CAD build for the part. Positions are in the model's coordinates, mm. Face numbers are marked on the shaded views. A direction names the side the tool comes from. Round coordinates to 2 decimals unless told otherwise and drop trailing zeros. Loops run counter-clockwise (first coordinate to the right, second up) from the corner with the lowest first, then second, coordinate; pieces in that order, holes last. Notation, with made-up numbers: (-21, -26.75) -> (11, -26.75) arc R27 ccw to (11, -9.75) -> close; hole circle Ø3 at (67.5, -8). An arc over 180 degrees is marked (long way). Answer as CSV lines item,"result".
```python
from build123d import *

# Parameters (mm, degrees)
SKETCH1_W                = 42.418
SKETCH1_H                = 0.006053875
SKETCH1_H_2              = 42.424053875
BOSS_EXTRUDE1_DEPTH      = 58.42
CUT_EXTRUDE3_DEPTH       = 68.58
SKETCH3_W                = 38.1
SKETCH3_H                = 15.367
SKETCH3_W_2              = 76.2
CUT_EXTRUDE4_DEPTH       = 77.078788463
BOSS_EXTRUDE6_DEPTH      = 3.302
BOSS_EXTRUDE6_DEPTH_BACK = 60
CUT_EXTRUDE9_DEPTH       = 106
SKETCH4_R                = 2.667
CUT_EXTRUDE6_DEPTH       = 106
CUT_EXTRUDE6_DEPTH_BACK  = 20
CUT_EXTRUDE13_DEPTH      = 106
SKETCH11_R               = 35
CUT_EXTRUDE15_DEPTH      = 106


with BuildPart() as part:
    # Sketch1 → Boss-Extrude1 (new body)
    with BuildSketch(Plane(origin=(0, 0, 0), x_dir=(1, 0, 0), z_dir=(0, 1, 0))):
        with BuildLine():
            ThreePointArc((36.658549334, 5.015053409), (0, 37), (-36.658549334, 5.015053409))
            Line((-36.658549334, 5.015053409), (-25.85615018, -105.598244919))
            ThreePointArc((-25.85615018, -105.598244919), (0, -129.052312238), (25.85615018, -105.598244919))
            Line((25.85615018, -105.598244919), (36.658549334, 5.015053409))
        make_face()
        with Locations((0, 21.205973063)):
            Rectangle(SKETCH1_W, SKETCH1_H, mode=Mode.SUBTRACT)
        with Locations((0, -21.212026937)):
            Rectangle(SKETCH1_W, SKETCH1_H, mode=Mode.SUBTRACT)
        with Locations((0, -45.723026938)):
            Rectangle(SKETCH1_W, SKETCH1_H_2, mode=Mode.SUBTRACT)
    extrude(amount=BOSS_EXTRUDE1_DEPTH)

    # Sketch2 → Cut-Extrude3 (cut)
    with BuildSketch(Plane(origin=(0, 58.42, 0), x_dir=(1, 0, 0), z_dir=(0, 1, 0))):
        with BuildLine():
            Line((-21.209, -66.935053875), (-17.681227978, -103.058371806))
            ThreePointArc((-17.681227978, -103.058371806), (0, -119.096981901), (17.681227978, -103.058371806))
            Line((17.681227978, -103.058371806), (21.209, -66.935053875))
            Line((21.209, -66.935053875), (-21.209, -66.935053875))
        make_face()
    extrude(amount=-CUT_EXTRUDE3_DEPTH, mode=Mode.SUBTRACT)

    # Sketch3 → Cut-Extrude4 (cut, through all)
    with BuildSketch(Plane(origin=(35.827089604, 0, 3.498842619), x_dir=(0.097196738, 0, -0.995265188), z_dir=(0.995265188, 0, 0.097196738))):
        with Locations((-121.635123595, 7.6835)):
            Rectangle(SKETCH3_W, SKETCH3_H)
        with Locations((-83.535123595, 7.6835)):
            Rectangle(SKETCH3_W, SKETCH3_H)
        with Locations((-102.585123595, 50.7365)):
            Rectangle(SKETCH3_W_2, SKETCH3_H)
    extrude(amount=-CUT_EXTRUDE4_DEPTH, mode=Mode.SUBTRACT)

    # Sketch7 → Boss-Extrude6 (add, two sides)
    with BuildSketch(Plane.XY.offset(21.209)) as boss_extrude6_sk:
        with BuildLine():
            Line((-34.93, 93.35), (-40.014696591, 94.207479888))
            Line((-40.014696591, 94.207479888), (-40.014696591, 55.40139672))
            Line((-40.014696591, 55.40139672), (41.480417685, 55.40139672))
            Line((41.480417685, 55.40139672), (41.480417685, 93.35))
            Line((41.480417685, 93.35), (34.93, 93.35))
            ThreePointArc((34.93, 93.35), (0, 58.42), (-34.93, 93.35))
        make_face()
    extrude(amount=BOSS_EXTRUDE6_DEPTH)
    extrude(boss_extrude6_sk.sketch, amount=-BOSS_EXTRUDE6_DEPTH_BACK)

    # Sketch9 → Cut-Extrude9 (cut)
    with BuildSketch(Plane.XZ):
        with BuildLine():
            Line((36.658549334, -5.015053409), (29.559345914, 67.678641264))
            Line((29.559345914, 67.678641264), (73.660631966, -15.324129582))
            Line((73.660631966, -15.324129582), (14.272065625, -84.211573711))
            Line((14.272065625, -84.211573711), (-60.028569558, -39.869360469))
            Line((-60.028569558, -39.869360469), (-30.128608249, 61.849567226))
            Line((-30.128608249, 61.849567226), (-36.658549334, -5.015053409))
            ThreePointArc((-36.658549334, -5.015053409), (0, -37), (36.658549334, -5.015053409))
        make_face()
    extrude(amount=-CUT_EXTRUDE9_DEPTH, mode=Mode.SUBTRACT)

    # Sketch4 → Cut-Extrude6 (cut, two sides)
    with BuildSketch(Plane(origin=(0, 58.42, 0), x_dir=(1, 0, 0), z_dir=(0, 1, 0))) as cut_extrude6_sk:
        with Locations((9.8, 0.389)):
            Circle(SKETCH4_R)
    extrude(amount=CUT_EXTRUDE6_DEPTH, mode=Mode.SUBTRACT)
    extrude(cut_extrude6_sk.sketch, amount=-CUT_EXTRUDE6_DEPTH_BACK, mode=Mode.SUBTRACT)

    # Sketch10 → Cut-Extrude13 (cut)
    with BuildSketch(Plane(origin=(35.827089604, 0, 3.498842619), x_dir=(0.097196738, 0, -0.995265188), z_dir=(0.995265188, 0, 0.097196738))):
        Polygon((-21.112119301, 84.442127612), (-21.112119301, 80.442127612), (1.82615742, 80.442127612), (48.352358454, 80.442127612), (47.215493026, 104.044705577), (-21.112119301, 100.753569315), align=None)
        Polygon((-34.412747442, 80.442127612), (-21.112119301, 80.442127612), (-21.112119301, 84.442127612), (-21.112119301, 100.753569315), (-34.412747442, 100.753569315), align=None)
    extrude(amount=-CUT_EXTRUDE13_DEPTH, mode=Mode.SUBTRACT)

    # Sketch11 → Cut-Extrude15 (cut)
    with BuildSketch(Plane(origin=(0, 58.42, 0), x_dir=(1, 0, 0), z_dir=(0, 1, 0))):
        Circle(SKETCH11_R)
    extrude(amount=CUT_EXTRUDE15_DEPTH, mode=Mode.SUBTRACT)


solid = part.part
```
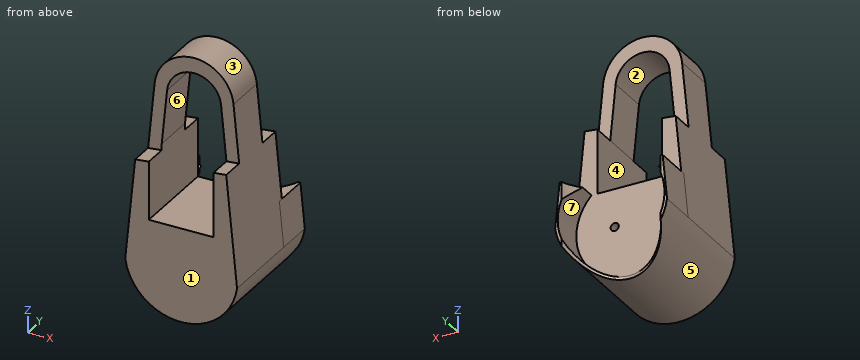
Q1. Slice it at D-D, the plane z = 56. Give the cut face in (x, y).
Results:
outline,"(-30.7, 0) -> (-21.21, 0) -> (-21.21, 58.42) -> (-30.7, 58.42) -> close; (21.21, 0) -> (30.7, 0) -> (30.7, 58.42) -> (21.21, 58.42) -> close"
Q2. Probe L1, parallel to Y at x = -17, z = 110.5; L2, parallel to X at y = 19, z = 105.5; L3, parallel to Z at x = 30, y = 59. List the from-to ranges inside material, lowest first. Write a range as [from, to].
Results:
L1,"[15.37, 43.05]"
L2,"[-25.87, -17.27], [17.27, 25.87]"
L3,"[-21.66, -18.03], [18.03, 24.51]"
Q3. Slice it at A-A, the plane z = 29. Give the cut face in (x, y), and give its area (3 significant figures).
Results:
outline,"(-33.34, 0) -> (-21.21, 0) -> (-21.21, 58.42) -> (-33.34, 58.42) -> close; (21.21, 0) -> (33.34, 0) -> (33.34, 58.42) -> (21.21, 58.42) -> close"
area,"1,420 mm2"
Q4. Slice it at B-B, the plane y = 8.5. Count the separate pieces of the cut face and the enclosed holes in it, and give its area (3 significant figures).
Results:
separate pieces,"1"
enclosed holes,"2"
area,"4,710 mm2"
Q5. Two-plate mould, pull along X, no slides. Class the marked faces 1, 2, 3 and 4: pulls with the +X half, pulls with the -X half, needs draft (parallel to the pull), parting line crosses it, or undercut.
Results:
face 1,"needs draft"
face 2,"undercut"
face 3,"parting line crosses it"
face 4,"undercut"
Q6. Drop flat-ended pins along their axis: pin 1 Ø2 at (y, z) = (21, 69) entering from +X; pin 2 Ø7 at (x, y) = (30.5, 68) entering from +Z; pin 3 Ø8 at (y, z) = (56.5, 47) entering from -X. Give the stop position or say it passes through.
Results:
pin 1,"x = 29.53"
pin 2,"z = 24.51"
pin 3,"x = -31.97"
Q7. Tool access for the marked faces 5, 6 and 7: list every direction of +Z, -Z, +X, -X, +Y, -Y with a clear straight run to the whole face (end or side of a thin tool).
Results:
face 5,"-Z, +Y, -Y"
face 6,"+Y, -Y"
face 7,"+Y"
